Input: part model. Units: mm. Frame: model coordinates. A direction names the side the tool comes from. Coordinates: 2 decimals unless noted, no trailing zeros. Loops run counter-clockwise (first coordinate to the right, second up) from the corner with the lowest first, then second, coordinate; pieces in that order, holes last. Notation, with made-up numbers: M -23,83 L 23,83 A24 cw 23,95 Z; hole C 88,63.25 d7. An arc over 180 degrees is marked long. Use a Markdown table: item, result. Add a question column.
1. Section D-D on x = -90. Output: boundary loops of the cut face in (y, z).
2. Draft query along X for faces 6 (the flat face through (6, 62, 3)), 7 (the flat face through (-200, 88, 3)), 8 (the cylindrical face through (-7, 49, 3)), 9 (the flat face through (-203, 25, 3)). Return one class per face: +X half, -X half, draft (parallel to the pull), parting line (faces both ways), or undercut.
3. Set-up query: faces 1 (the flat face through (-203, 100, 3)), 2 (the flat face through (-101, 0, 3)), 3 (the flat face through (-195, 175, 3)), 4 (the flat face through (-17, 142, 3)), 5 (the flat face through (3, 75, 3)). Return all of +Z, -Z, +X, -X, +Y, -Y with unobstructed straight access to the full face (end or side cutting, diameter ignored); none if empty.
4. Section A-A on y = 80. Output: boundary loops of the cut face in (x, z), then the cut area to 3 significant figures.
5. Pin query (flat end, axial travel): pin 1 (1.8 mm diameter, centred on y = 127, z = 2.5, fed in from -X); pin 2 (1.8 mm diameter, centred on y = 133, z = 2, fed in from +X); pin 3 (1.5 mm diameter, centred on x = -19, z = 2, fed in from +Y). Return the tip coordinate at first contact, or that it passes through.
6. Section B-B on x = -10. Output: boundary loops of the cut face in (y, z).
7. Section C-C on z = 1.25. State how many separate pieces and enclosed holes the cut face has, then the cut area to 3 significant figures.
8. Line query: L1, parallel to Y at x = -190, z = 3.5; L2, parallel to X at y = 126, z = 2.3; L3, parallel to X at y = 97.5, z = 4.8. Output: solid intervals per line, ascending. Write a range as [from, to].
```python
from build123d import *

# Parameters (mm, degrees)
BOSS_EXTRUDE1_DEPTH   = 6
SKETCH2_W             = 6
SKETCH2_H             = 25
BOSS_EXTRUDE2_DEPTH   = 6
LPATTERN1_OUTLINE_W   = 6
LPATTERN1_OUTLINE_H   = 6
LPATTERN1_DEPTH       = 25
LPATTERN1_START       = 50
LPATTERN1_2_OUTLINE_W = 6
LPATTERN1_2_OUTLINE_H = 6
LPATTERN1_2_DEPTH     = 25
LPATTERN1_START_2     = 100
LPATTERN1_3_OUTLINE_W = 6
LPATTERN1_3_OUTLINE_H = 6
LPATTERN1_3_DEPTH     = 25
LPATTERN1_START_3     = 150
LPATTERN1_4_OUTLINE_W = 6
LPATTERN1_4_OUTLINE_H = 6
LPATTERN1_4_DEPTH     = 25
SKETCH5_R             = 5
CUT_EXTRUDE1_DEPTH    = 271.364568685
SKETCH6_W             = 5
SKETCH6_H             = 65
CUT_EXTRUDE2_DEPTH    = 10


# Read off the part's stored shape, not the designer's step: LPattern1
with BuildPart() as part:
    # Sketch1 → Boss-Extrude1 (new body)
    with BuildSketch(Plane.XY):
        with BuildLine():
            Line((-178, 175), (-200, 175))
            Line((-200, 175), (-200, 0))
            Line((-200, 0), (0, 0))
            Line((0, 0), (0, 175))
            Line((0, 175), (-22, 175))
            Line((-22, 175), (-22, 110))
            ThreePointArc((-22, 110), (-31.037807258, 73.555302549), (-56.056819802, 45.55625))
            ThreePointArc((-56.056819802, 45.55625), (-100, 27.5), (-143.943180198, 45.55625))
            ThreePointArc((-143.943180198, 45.55625), (-168.962192742, 73.555302549), (-178, 110))
            Line((-178, 110), (-178, 175))
        make_face()
    extrude(amount=BOSS_EXTRUDE1_DEPTH)

    # Sketch2 → Boss-Extrude2 (add)
    with BuildSketch(Plane.XY.offset(6)):
        with Locations((-203, 162.5)):
            Rectangle(SKETCH2_W, SKETCH2_H)
    extrude(amount=-BOSS_EXTRUDE2_DEPTH)

    # LPattern1 outline → LPattern1 (add)
    with BuildSketch(Plane(origin=(0, 0, 0), x_dir=(1, 0, 0), z_dir=(0, 1, 0))):
        with Locations((-203, -3)):
            Rectangle(LPATTERN1_OUTLINE_W, LPATTERN1_OUTLINE_H)
        with Locations((3, -3)):
            Rectangle(LPATTERN1_OUTLINE_W, LPATTERN1_OUTLINE_H)
    extrude(amount=LPATTERN1_DEPTH)

    # LPattern1 2 outline → LPattern1 2 (add)
    with BuildSketch(Plane(origin=(0, 0, 0), x_dir=(1, 0, 0), z_dir=(0, 1, 0)).offset(LPATTERN1_START)):
        with Locations((-203, -3)):
            Rectangle(LPATTERN1_2_OUTLINE_W, LPATTERN1_2_OUTLINE_H)
        with Locations((3, -3)):
            Rectangle(LPATTERN1_2_OUTLINE_W, LPATTERN1_2_OUTLINE_H)
    extrude(amount=LPATTERN1_2_DEPTH)

    # LPattern1 3 outline → LPattern1 3 (add)
    with BuildSketch(Plane(origin=(0, 0, 0), x_dir=(1, 0, 0), z_dir=(0, 1, 0)).offset(LPATTERN1_START_2)):
        with Locations((-203, -3)):
            Rectangle(LPATTERN1_3_OUTLINE_W, LPATTERN1_3_OUTLINE_H)
        with Locations((3, -3)):
            Rectangle(LPATTERN1_3_OUTLINE_W, LPATTERN1_3_OUTLINE_H)
    extrude(amount=LPATTERN1_3_DEPTH)

    # LPattern1 4 outline → LPattern1 4 (add)
    with BuildSketch(Plane(origin=(0, 0, 0), x_dir=(1, 0, 0), z_dir=(0, 1, 0)).offset(LPATTERN1_START_3)):
        with Locations((3, -3)):
            Rectangle(LPATTERN1_4_OUTLINE_W, LPATTERN1_4_OUTLINE_H)
    extrude(amount=LPATTERN1_4_DEPTH)

    # Sketch5 → Cut-Extrude1 (cut, through all)
    with BuildSketch(Plane.XY.offset(6)):
        with Locations((-10, 45)):
            Circle(SKETCH5_R)
        with Locations(Location((-190, 45, 0), (0, 0, 180))):
            Circle(SKETCH5_R)
    extrude(amount=-CUT_EXTRUDE1_DEPTH, mode=Mode.SUBTRACT)

    # Sketch6 → Cut-Extrude2 (cut)
    with BuildSketch(Plane.XY.offset(6)):
        with Locations((-180.5, 142.5)):
            Rectangle(SKETCH6_W, SKETCH6_H)
        with Locations((-19.5, 142.5)):
            Rectangle(SKETCH6_W, SKETCH6_H)
    extrude(amount=-CUT_EXTRUDE2_DEPTH, mode=Mode.SUBTRACT)


solid = part.part
```
Answers below:
| question | item | result |
|---|---|---|
| 1 | outline | M 0,0 L 28.31,0 L 28.31,6 L 0,6 Z |
| 2 | face 6 | +X half |
| 2 | face 7 | -X half |
| 2 | face 8 | undercut |
| 2 | face 9 | draft |
| 3 | face 1 | +Z, -Z, -X |
| 3 | face 2 | +Z, -Z, +X, -X, -Y |
| 3 | face 3 | +Z, -Z, +X, -X, +Y |
| 3 | face 4 | +Z, -Z, +Y |
| 3 | face 5 | +Z, -Z, +X |
| 4 | outline | M -200,0 L -172,0 L -172,6 L -200,6 Z; M -28,0 L 0,0 L 0,6 L -28,6 Z |
| 4 | area | 336 mm² |
| 5 | pin 1 | stops at x = -200 |
| 5 | pin 2 | stops at x = 0 |
| 5 | pin 3 | stops at y = 110 |
| 6 | outline | M 0,0 L 40,0 L 40,6 L 0,6 Z; M 50,0 L 175,0 L 175,6 L 50,6 Z |
| 7 | separate pieces | 1 |
| 7 | enclosed holes | 2 |
| 7 | area | 15,400 mm² |
| 8 | L1 | y = [0, 40], [50, 175] |
| 8 | L2 | x = [-200, -183], [-17, 0] |
| 8 | L3 | x = [-200, -176.99], [-23.01, 0] |
